```python
from build123d import *

# Parameters (mm, degrees)
SKETCH1_W           = 15
SKETCH1_H           = 11.5
BOSS_EXTRUDE1_DEPTH = 17.3
SKETCH2_W           = 13
SKETCH2_H           = 10.5
CUT_EXTRUDE1_DEPTH  = 26.62303651
FILLET1_R           = 1
SKETCH7_W           = 1.5
SKETCH7_H           = 8.5
BOSS_EXTRUDE4_DEPTH = 3
BOSS_EXTRUDE5_DEPTH = 3
BOSS_EXTRUDE6_DEPTH = 3
CUT_EXTRUDE4_DEPTH  = 29.32141416
CUT_EXTRUDE5_DEPTH  = 2
FILLET6_START       = -16.47329
FILLET6_DEPTH       = 0.536538654
FILLET6_START_2     = -10.163248654
FILLET6_2_DEPTH     = 0.536538654
FILLET6_START_3     = -11.029274158
FILLET6_3_DEPTH     = 2.229274158
FILLET6_START_4     = -17.3
FILLET6_4_DEPTH     = 2.229274058
FILLET6_START_5     = 3
FILLET6_5_DEPTH     = 3


with BuildPart() as part:
    # Sketch1 → Boss-Extrude1 (new body)
    with BuildSketch(Plane.XY):
        with Locations((7.5, 5.75)):
            Rectangle(SKETCH1_W, SKETCH1_H)
    extrude(amount=-BOSS_EXTRUDE1_DEPTH)

    # Sketch2 → Cut-Extrude1 (cut, through all)
    with BuildSketch(Plane.XY):
        with Locations((7.5, 5.25)):
            Rectangle(SKETCH2_W, SKETCH2_H)
    extrude(amount=-CUT_EXTRUDE1_DEPTH, mode=Mode.SUBTRACT)

    # Fillet1
    fillet1_edges = [part.edges().sort_by_distance(p)[0] for p in [
        (1, 10.5, -8.65),
        (14, 10.5, -8.65),
    ]]
    fillet(fillet1_edges, radius=FILLET1_R)

    # Sketch7 → Boss-Extrude4 (add)
    with BuildSketch(Plane.XZ):
        with Locations((-0.75, -13.05)):
            Rectangle(SKETCH7_W, SKETCH7_H)
        with Locations((15.75, -13.05)):
            Rectangle(SKETCH7_W, SKETCH7_H)
    extrude(amount=-BOSS_EXTRUDE4_DEPTH)

    # Sketch11 → Boss-Extrude5 (add)
    with BuildSketch(Plane.XZ):
        with BuildLine():
            Line((-1.5, -8.8), (-1.5, -17.3))
            ThreePointArc((-1.5, -17.3), (-5.75, -13.05), (-1.5, -8.8))
        make_face()
    extrude(amount=-BOSS_EXTRUDE5_DEPTH)

    # Sketch12 → Boss-Extrude6 (add)
    with BuildSketch(Plane.XZ):
        with BuildLine():
            Line((14, 0), (14, -17.3))
            Line((14, -17.3), (16.5, -17.3))
            ThreePointArc((16.5, -17.3), (20.75, -13.05), (16.5, -8.8))
            Line((16.5, -8.8), (15, -8.8))
            Line((15, -8.8), (15, 0))
            Line((15, 0), (14, 0))
        make_face()
    extrude(amount=-BOSS_EXTRUDE6_DEPTH)

    # Sketch13 → Cut-Extrude4 (cut, through all)
    with BuildSketch(Plane(origin=(0, 3, 0), x_dir=(1, 0, 0), z_dir=(0, 1, 0))):
        with BuildLine():
            Line((-0.25, 12.3), (-1.5, 12.3))
            ThreePointArc((-1.5, 12.3), (-2.25, 13.05), (-1.5, 13.8))
            Line((-1.5, 13.8), (-0.25, 13.8))
            ThreePointArc((-0.25, 13.8), (0.5, 13.05), (-0.25, 12.3))
        make_face()
        with BuildLine():
            Line((15.25, 13.8), (16.5, 13.8))
            ThreePointArc((16.5, 13.8), (17.25, 13.05), (16.5, 12.3))
            Line((16.5, 12.3), (15.25, 12.3))
            ThreePointArc((15.25, 12.3), (14.5, 13.05), (15.25, 13.8))
        make_face()
    extrude(amount=-CUT_EXTRUDE4_DEPTH, mode=Mode.SUBTRACT)

    # Sketch14 → Cut-Extrude5 (cut)
    with BuildSketch(Plane(origin=(0, 3, 0), x_dir=(1, 0, 0), z_dir=(0, 1, 0))):
        Polygon((-1.5, 15.936751346), (-4, 14.493375673), (-4, 11.606624327), (-1.5, 10.163248654), (1, 11.606624327), (1, 14.493375673), align=None)
        Polygon((16.5, 15.936751346), (14, 14.493375673), (14, 11.606624327), (16.5, 10.163248654), (19, 11.606624327), (19, 14.493375673), align=None)
    extrude(amount=-CUT_EXTRUDE5_DEPTH, mode=Mode.SUBTRACT)

    # Fillet6: read off the stored shape, not the designer's step
    # Fillet6 outline → Fillet6 (add)
    with BuildSketch(Plane.XY.offset(FILLET6_START)):
        with BuildLine():
            ThreePointArc((17, 3), (15.585786438, 3.585786438), (15, 5))
            Line((15, 5), (15, 3))
            Line((15, 3), (17, 3))
        make_face()
        with BuildLine():
            ThreePointArc((0, 5), (-0.585786438, 3.585786438), (-2, 3))
            Line((-2, 3), (0, 3))
            Line((0, 3), (0, 5))
        make_face()
    extrude(amount=FILLET6_DEPTH)

    # Fillet6 2 outline → Fillet6 2 (add)
    with BuildSketch(Plane.XY.offset(FILLET6_START_2)):
        with BuildLine():
            ThreePointArc((17, 3), (15.585786438, 3.585786438), (15, 5))
            Line((15, 5), (15, 3))
            Line((15, 3), (17, 3))
        make_face()
        with BuildLine():
            ThreePointArc((0, 5), (-0.585786438, 3.585786438), (-2, 3))
            Line((-2, 3), (0, 3))
            Line((0, 3), (0, 5))
        make_face()
    extrude(amount=FILLET6_2_DEPTH)

    # Fillet6 3 outline → Fillet6 3 (add)
    with BuildSketch(Plane.XY.offset(FILLET6_START_3)):
        with BuildLine():
            ThreePointArc((17, 3), (15.585786438, 3.585786438), (15, 5))
            Line((15, 5), (15, 3))
            Line((15, 3), (17, 3))
        make_face()
        with BuildLine():
            ThreePointArc((0, 5), (-0.585786438, 3.585786438), (-2, 3))
            Line((-2, 3), (0, 3))
            Line((0, 3), (0, 5))
        make_face()
    extrude(amount=FILLET6_3_DEPTH)

    # Fillet6 4 outline → Fillet6 4 (add)
    with BuildSketch(Plane.XY.offset(FILLET6_START_4)):
        with BuildLine():
            ThreePointArc((17, 3), (15.585786438, 3.585786438), (15, 5))
            Line((15, 5), (15, 3))
            Line((15, 3), (17, 3))
        make_face()
        with BuildLine():
            ThreePointArc((0, 5), (-0.585786438, 3.585786438), (-2, 3))
            Line((-2, 3), (0, 3))
            Line((0, 3), (0, 5))
        make_face()
    extrude(amount=FILLET6_4_DEPTH)

    # Fillet6 5 outline → Fillet6 5 (cut)
    with BuildSketch(Plane(origin=(0, 0, 0), x_dir=(1, 0, 0), z_dir=(0, 1, 0)).offset(FILLET6_START_5)):
        Polygon((16.5, 15.936751346), (15, 15.070725942), (17, 15.070725942), (17, 15.648076211), align=None)
        with BuildLine():
            ThreePointArc((17, 8.829514246), (16.750435167, 8.807384978), (16.5, 8.8))
            Line((16.5, 8.8), (17, 8.8))
            Line((17, 8.8), (17, 8.829514246))
        make_face()
        with BuildLine():
            Line((17, 17.3), (16.5, 17.3))
            ThreePointArc((16.5, 17.3), (16.750435167, 17.292615022), (17, 17.270485754))
            Line((17, 17.270485754), (17, 17.3))
        make_face()
        with BuildLine():
            Line((-2, 17.3), (-2, 17.270485754))
            ThreePointArc((-2, 17.270485754), (-1.750435167, 17.292615022), (-1.5, 17.3))
            Line((-1.5, 17.3), (-2, 17.3))
        make_face()
        Polygon((-1.5, 15.936751346), (-2, 15.648076211), (-2, 15.070725942), (0, 15.070725942), align=None)
        Polygon((-2, 11.029274158), (-2, 10.451923789), (-1.5, 10.163248654), (0, 11.029274058), align=None)
        with BuildLine():
            ThreePointArc((-1.5, 8.8), (-1.750435167, 8.807384978), (-2, 8.829514246))
            Line((-2, 8.829514246), (-2, 8.8))
            Line((-2, 8.8), (-1.5, 8.8))
        make_face()
        Polygon((17, 11.029274158), (15, 11.029274158), (16.5, 10.163248654), (17, 10.451923789), align=None)
    extrude(amount=FILLET6_5_DEPTH, mode=Mode.SUBTRACT)


solid = part.part
```
Geometry: final body of the model. Coordinates: model frame, mm. A direction names the side the tool comes from. Give positions to 0.01 mm unless a question says otherwise; leave off trailing zeros. Write each loop counter-clockwise with the first axis right and the second up, starting at its lowest first coordinate (ties: lowest second). Pieces come first, ordered by that corner, then holes.
1. Section query B-B, the plane y = 7. Return loops of the section in (x, z).
2. Section query C-C, the plane z = -3. Return loops of the section in (x, y), then the cut area to 3 significant figures.
3. Pin query (flat end, axial travel): P1, Ø3, axis at y = 1.5, z = -6.5, coming from the +X side; P2, Ø6, axis at y = 4.5, z = -15, coming from the -X side; P3, Ø1.1, axis at x = 19.5, z = -12.5, coming from the +Y side; P4, Ø3, axis at y = 9, z = -7.5, coming from the -X side. Return the tip coordinate at first contact, or that it passes through.
4. Line query: probe 1 along X at (y, z) = (7.75, -2); probe 2 along Y at (x, z) = (15.5, -11); probe 3 along X at (y, z) = (1.5, -15.5). Output: solid intervals per line, ascending.
5. Reachability of faces 1 (the flat face through (19.3, 3, -13)), 2 (the cylindrical face through (1.285, 10.199, -8.771)), 3 (the flat face through (14.5, 3, -13.1)), 4 (the cylindrical face through (-2.25, 0.51, -13.03)) from +Z, -Z, +X, -X, +Y, -Y: full face, straight path, thin tool, end or side. Return the list, or none.
6. Section query D-D, the plane x = 9.75. Return loops of the section in (y, z).
7. Draft query along Z for faces 5 (the flat face through (15.9, 0.5, -12.3)), 6 (the cylindrical face through (13.715, 10.199, -8.771)), 7 (the flat face through (0.5, 3, -13.1)), 8 (the flat face through (6, 11, 0)). Return one class per face: released by +Z, released by -Z, zero draft, split by the parting line, or undercut.
8. Section query A-A, the plane z = -13.05. Count the separate pieces of the cut face and the enclosed holes in it, then the cut area to 3 significant figures.
Computed:
1. outline: (0, -17.3) - (1, -17.3) - (1, 0) - (0, 0) - close; (14, -17.3) - (15, -17.3) - (15, 0) - (14, 0) - close
2. outline: (0, 0) - (1, 0) - (1, 9.5) arc R1 cw to (2, 10.5) - (13, 10.5) arc R1 cw to (14, 9.5) - (14, 0) - (15, 0) - (15, 11.5) - (0, 11.5) - close
2. area: 36.4 mm2
3. P1: stops at x = 15
3. P2: stops at x = -5.75
3. P3: stops at y = 3
3. P4: stops at x = 0
4. probe 1: x = 0 to 1, 14 to 15
4. probe 2: y = 0 to 1
4. probe 3: x = -4.97 to -2.26, -0.74 to 1, 14 to 15.74, 17.26 to 19.97
5. face 1: +Z, -Z, +X, +Y
5. face 2: +Z, -Z, -Y
5. face 3: none
5. face 4: +Y, -Y
6. outline: (10.5, -17.3) - (11.5, -17.3) - (11.5, 0) - (10.5, 0) - close
7. face 5: undercut
7. face 6: zero draft
7. face 7: undercut
7. face 8: released by +Z
8. separate pieces: 5
8. enclosed holes: 0
8. area: 45.4 mm2
